from build123d import *

# Parameters (mm, degrees)
SKETCH_1_W      = 52
SKETCH_1_H      = 29
SKETCH_1_R      = 2
EXTRUDE_1_DEPTH = 2
SKETCH_2_W      = 18
SKETCH_2_H      = 16
EXTRUDE_2_DEPTH = 2
SKETCH_3_W      = 38.5
SKETCH_3_H      = 3
EXTRUDE_3_DEPTH = 9


with BuildPart() as part:
    # 草图1 → 凸台-拉伸1 (new body)
    with BuildSketch(Plane(origin=(0, 0, 0), x_dir=(1, 0, 0), z_dir=(0, 1, 0))):
        with Locations((26, 14.5)):
            Rectangle(SKETCH_1_W, SKETCH_1_H)
        with Locations(Location((49.5, 26.5, 0), (0, 0, 270))):
            Circle(SKETCH_1_R, mode=Mode.SUBTRACT)
        with Locations(Location((49.5, 2.5, 0), (0, 0, 90))):
            Circle(SKETCH_1_R, mode=Mode.SUBTRACT)
        with Locations(Location((2.5, 2.5, 0), (0, 0, 270))):
            Circle(SKETCH_1_R, mode=Mode.SUBTRACT)
        with Locations(Location((2.5, 26.5, 0), (0, 0, 90))):
            Circle(SKETCH_1_R, mode=Mode.SUBTRACT)
    extrude(amount=EXTRUDE_1_DEPTH)

    # 草图2 → 凸台-拉伸2 (add)
    with BuildSketch(Plane(origin=(0, 2, 0), x_dir=(1, 0, 0), z_dir=(0, 1, 0))):
        with Locations((36.2, 14.5)):
            Rectangle(SKETCH_2_W, SKETCH_2_H)
    extrude(amount=EXTRUDE_2_DEPTH)

    # 草图3 → 凸台-拉伸3 (add)
    with BuildSketch(Plane.XZ):
        with Locations((27.75, -1.5)):
            Rectangle(SKETCH_3_W, SKETCH_3_H)
        with Locations((27.75, -27.5)):
            Rectangle(SKETCH_3_W, SKETCH_3_H)
    extrude(amount=EXTRUDE_3_DEPTH)


solid = part.part
Part model, mm, in its own coordinate system. A direction names the side the tool comes from. Give positions to 0.01 mm unless a question says otherwise; leave off trailing zeros. Write each loop counter-clockwise with the first axis right and the second up, starting at its lowest first coordinate (ties: lowest second). Pieces come first, ordered by that corner, then holes.
1) Cut at A-A on x = 49.5. Write the cut outline in (y, z), then the cut area to 3 significant figures.
Resolved:
outline: (0, -29) - (2, -29) - (2, -28.5) - (0, -28.5) - close; (0, -24.5) - (2, -24.5) - (2, -4.5) - (0, -4.5) - close; (0, -0.5) - (2, -0.5) - (2, 0) - (0, 0) - close
area: 42.0 mm2
2) Cut at B-B on y = -0.5. Write the cut outline in (x, z).
Resolved:
outline: (8.5, -29) - (47, -29) - (47, -26) - (8.5, -26) - close; (8.5, -3) - (47, -3) - (47, 0) - (8.5, 0) - close
3) Cut at D-D on x = 28.5. Write the cut outline in (y, z), then the cut area to 3 significant figures.
Resolved:
outline: (-9, -29) - (2, -29) - (2, -22.5) - (4, -22.5) - (4, -6.5) - (2, -6.5) - (2, 0) - (-9, 0) - (-9, -3) - (0, -3) - (0, -26) - (-9, -26) - close
area: 144 mm2
4) Cut at C-C on z = -26.5. Write the cut outline in (x, y), then the cut area to 4 significant figures.
Resolved:
outline: (0, 0) - (0.5, 0) - (0.5, 2) - (0, 2) - close; (4.5, 0) - (8.5, 0) - (8.5, -9) - (47, -9) - (47, 0) - (47.5, 0) - (47.5, 2) - (4.5, 2) - close; (51.5, 0) - (52, 0) - (52, 2) - (51.5, 2) - close
area: 434.5 mm2
5) Pin check, flat tips, straight feed: pin 1 (2.5 mm diameter, centred on x = 49.5, z = -26.5, fed in from -Y); pin 2 (1 mm diameter, centred on x = 10.5, y = -3.5, fed in from +Z); pin 3 (1.6 mm diameter, centred on x = 35.5, y = 3, fed in from +Z); pin 4 (0.9 mm diameter, centred on y = -4, z = -1.5, fed in from -X). Stop position of each tip, or through.
Resolved:
pin 1: passes through
pin 2: stops at z = 0
pin 3: stops at z = -6.5
pin 4: stops at x = 8.5
6) Two-plate mould, pull along Z, no slides. Class faces 4 (the face through (8.5, -4, -2)), 5 (the face through (27, -4, -3)), 6 (the face through (36, 3, -6.5)): released by +Z, released by -Z, zero draft, split by the parting line, or undercut.
Resolved:
face 4: zero draft
face 5: undercut
face 6: released by +Z
7) Probe L1, parallel to X at y = 1, z = -26.5; L2, parallel to Z at x = 45.5, y = -1; L3, parallel to Y at x = 24, z = -8.25. List the from-to ranges inside material, lowest first.
Resolved:
L1: x = 0 to 0.5, 4.5 to 47.5, 51.5 to 52
L2: z = -29 to -26, -3 to 0
L3: y = 0 to 2
8) Which spindle directions (+Z, -Z, +X, -X, +Y, -Y) get a long thin tool onto all of the face, cutting with end or side? Do faces 1 (the face through (27, -4, -26)), 2 (the face through (47, -4, -2)), 3 (the face through (8.5, -4, -28)). Say none if no direction does.
Resolved:
face 1: +X, -X, -Y
face 2: +Z, -Z, +X, -Y
face 3: +Z, -Z, -X, -Y
